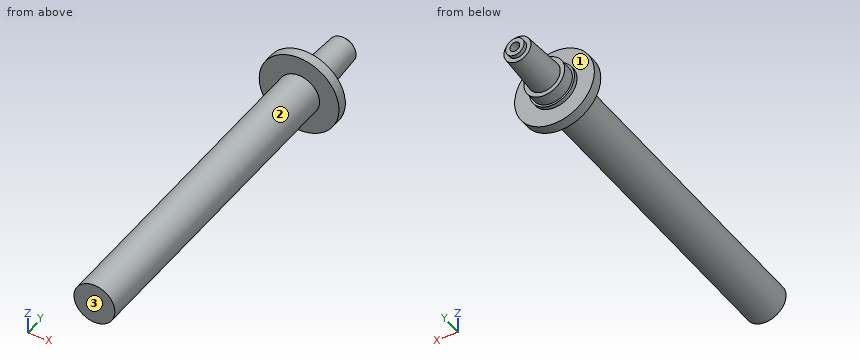
from build123d import *

# Parameters (mm, degrees)
SKETCH2_R           = 5.5
BOSS_EXTRUDE1_DEPTH = 1


with BuildPart() as part:
    # Sketch1 → Revolve1 (revolve)
    with BuildSketch(Plane.XY, mode=Mode.PRIVATE) as revolve1_sk:
        Polygon((0, 0), (5, 0), (5, 80), (9.75, 80), (9.75, 82.5), (5, 82.5), (5, 86.5), (3.9, 86.5), (3.3, 97), (2.25, 97), (2.25, 98), (1.2, 98), (1.2, 92), (0, 92), align=None)
    revolve(revolve1_sk.sketch.rotate(Axis((0, 92, 0), (0, -1, 0)), 180), axis=Axis((0, 92, 0), (0, -1, 0)))

    # Sketch2 → Boss-Extrude1 (add)
    with BuildSketch(Plane(origin=(0, 82.5, 0), x_dir=(1, 0, 0), z_dir=(0, 1, 0))):
        Circle(SKETCH2_R)
    extrude(amount=BOSS_EXTRUDE1_DEPTH)


solid = part.part
Model file for the job. Use its own axes, mm. Face numbers are marked on the shaded views. A direction names the side the tool comes from. Round coordinates to 2 decimals unless told otherwise and drop trailing zeros. Order: outer loops, then holes, each group sorted by start corner. A loop starts at its lowest first (then second) coordinate and runs counter-clockwise, first axis right, second up. Notation, with made-up numbers: M -32.5,78 L 5.5,78 A19 ccw 5.5,115 Z; hole C -6,87.25 d11. An arc over 180 degrees is marked long. Write each question's results on one line, items separated by ' | '. Start each with the question number.
(1) Which spindle directions (+Z, -Z, +X, -X, +Y, -Y) get a long thin tool onto all of the face, cutting with end or side? Do the marked faces 1, 2 and 3. Say none if no direction does.
(2) Saw through at A-A, the plane z = 0. Give the cut face in (x, y), then the cut area to 3 significant figures.
(3) Probe probe 1 along Y at (x, z) = (-1.5, 2.75); probe 2 along Y at (x, z) = (-5.5, -7); probe 3 along Z at (x, y) = (0, 94.1). List the from-to ranges inside material, lowest first. Write a range as from..to.
(4) Saw through at C-C, the plane y = 45.5. Give the cut face in (x, z).
(5) Drop flat-ended pins along their axis: pin 1 (10 mm diameter, centred on x = -7.5, y = 24.5, fed in from +Z); pin 2 (10 mm diameter, centred on x = 5, y = 45, fed in from -Z); pin 3 (1.5 mm diameter, centred on x = 4, y = 30, fed in from +Z). Give the stop position or say it passes through.
(6) Saw through at B-B, the plane x = 0. Give the cut face in (y, z), then the cut area to 3 significant figures.
(7) Saw through at D-D, the plane x = -8.5. Give the cut face in (y, z).
Established:
1) face 1: +Y | face 2: -Y | face 3: +Z, -Z, +X, -X, -Y
2) outline: M -9.75,80 L -5,80 L -5,0 L 5,0 L 5,80 L 9.75,80 L 9.75,82.5 L 5.5,82.5 L 5.5,83.5 L 5,83.5 L 5,86.5 L 3.9,86.5 L 3.3,97 L 2.25,97 L 2.25,98 L 1.2,98 L 1.2,92 L -1.2,92 L -1.2,98 L -2.25,98 L -2.25,97 L -3.3,97 L -3.9,86.5 L -5,86.5 L -5,83.5 L -5.5,83.5 L -5.5,82.5 L -9.75,82.5 Z | area: 955 mm^2
3) probe 1: y = 0..97 | probe 2: y = 80..82.5 | probe 3: z = -3.47..-1.2, 1.2..3.47
4) outline: C 0,0 d10
5) pin 1: stops at z = 4.33 | pin 2: stops at z = -5 | pin 3: stops at z = 3.8
6) outline: M 0,-5 L 80,-5 L 80,-9.75 L 82.5,-9.75 L 82.5,-5.5 L 83.5,-5.5 L 83.5,-5 L 86.5,-5 L 86.5,-3.9 L 97,-3.3 L 97,-2.25 L 98,-2.25 L 98,-1.2 L 92,-1.2 L 92,1.2 L 98,1.2 L 98,2.25 L 97,2.25 L 97,3.3 L 86.5,3.9 L 86.5,5 L 83.5,5 L 83.5,5.5 L 82.5,5.5 L 82.5,9.75 L 80,9.75 L 80,5 L 0,5 Z | area: 955 mm^2
7) outline: M 80,-4.78 L 82.5,-4.78 L 82.5,4.78 L 80,4.78 Z
